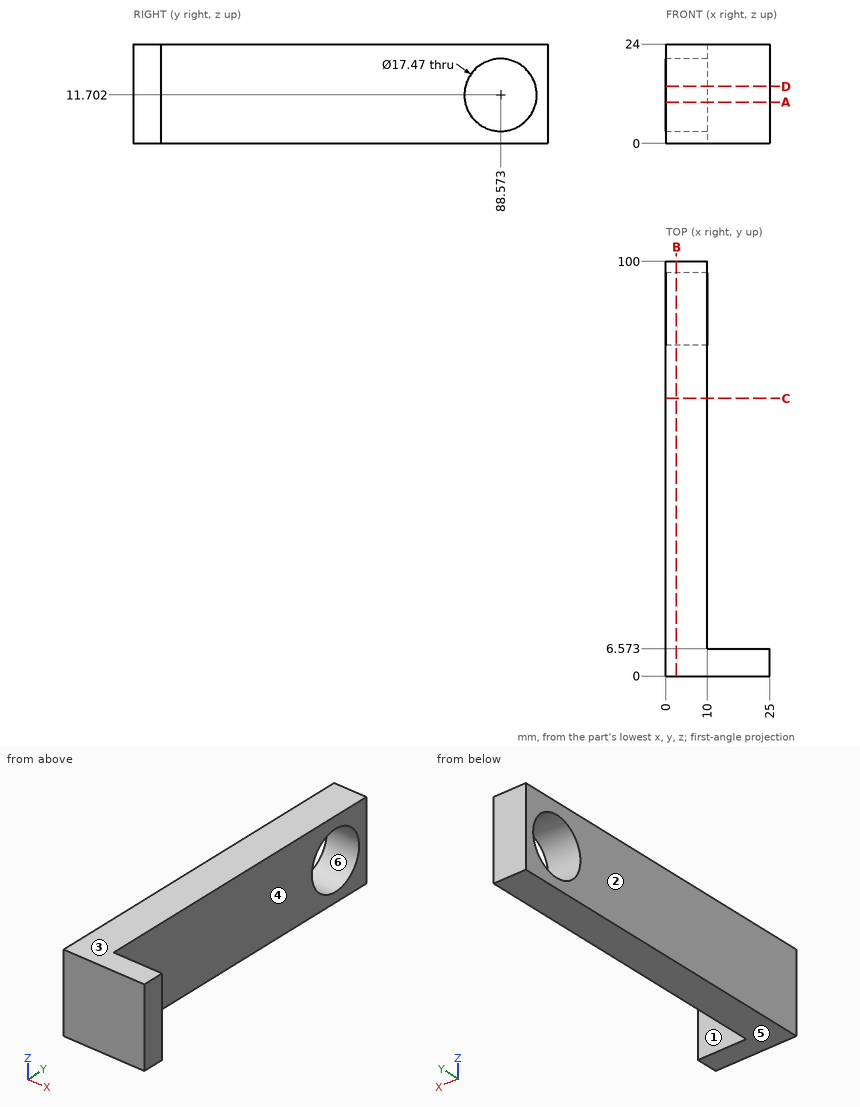
Drawing for the job (mm, zero at the part's lowest x, y, z). A direction names the side the tool comes from. Give positions to 0.01 mm unless a question says otherwise; leave off trailing zeros. Loops run counter-clockwise (first coordinate to the right, second up) from the corner with the lowest first, then second, coordinate; pieces in that order, holes last.
(1) Band-saw the part on B-B (x = 2.5). Write the cut outline in (y, z) (1 decimal), and give its area (3 significant figures).
Return value:
outline: (0, 0) - (100, 0) - (100, 24) - (0, 24) - close; hole circle Ø17.5 at (88.6, 11.7)
area: 2,160 mm2
(2) Band-saw the part on D-D (z = 13.75). Write the cut outline in (x, y) (1 decimal).
Return value:
outline: (0, 0) - (25, 0) - (25, 6.6) - (10, 6.6) - (10, 80.1) - (0, 80.1) - close; (0, 97.1) - (10, 97.1) - (10, 100) - (0, 100) - close
(3) Pull direction Z, two halves, no side cores. Call the marked faces 3, 4, 5 and 6: pulls with the +Z half, pulls with the -Z half, needs draft (parallel to the pull), parting line crosses it, or undercut.
Return value:
face 3: pulls with the +Z half
face 4: needs draft
face 5: pulls with the -Z half
face 6: undercut
(4) Band-saw the part on C-C (y = 67). Write the cut outline in (x, z), and give its area (3 significant figures).
Return value:
outline: (0, 0) - (10, 0) - (10, 24) - (0, 24) - close
area: 240 mm2
(5) Pin check, flat tips, straight feed: pin 1 (5 mm diameter, centred on x = 21.5, z = 13, fed in from +Y); pin 2 (7 mm diameter, centred on y = 74, z = 15.5, fed in from +X). Stop position of each tip, or through.
Return value:
pin 1: stops at y = 6.57
pin 2: stops at x = 10
(6) Drill centre lines: line 1 along X through (y, z) = (19, 3.5); line 2 along Y through (x, z) = (21.5, 3.25); line 3 along Z through (x, y) = (4, 84.5) (1 decimal). Where is each one in solid material? Low to high.
Return value:
line 1: x = 0 to 10
line 2: y = 0 to 6.57
line 3: z = 0 to 4, 19.4 to 24
(7) Band-saw the part on A-A (z = 10). Write the cut outline in (x, y) (1 decimal).
Return value:
outline: (0, 0) - (25, 0) - (25, 6.6) - (10, 6.6) - (10, 80) - (0, 80) - close; (0, 97.1) - (10, 97.1) - (10, 100) - (0, 100) - close
(8) 3-axis set-ups, long thin cutter, end or side, ignore diameter. For the marked faces 1 and 2: which of +Z, -Z, +X, -X, +Y, -Y reach the whole face in a straight line?
Return value:
face 1: +Z, -Z, +X, +Y
face 2: +Z, -Z, -X, +Y, -Y
